Job drawing, mm, ordinate dimensions from the low corner. One solid piece. A direction names the side the tool comes from. Round coordinates to 2 decimals unless told otherwise and drop trailing zeros. Loops run counter-clockwise (first coordinate to the right, second up) from the corner with the lowest first, then second, coordinate; pieces in that order, holes last. Notation, with made-up numbers: (33.5, 37) - (57.5, 37) arc R17 cw to (57.5, 54) - close; hole circle Ø1 at (27.25, 16). An arc over 180 degrees is marked (long way). One line per question, with ' | ' between items. Start each with the question number.
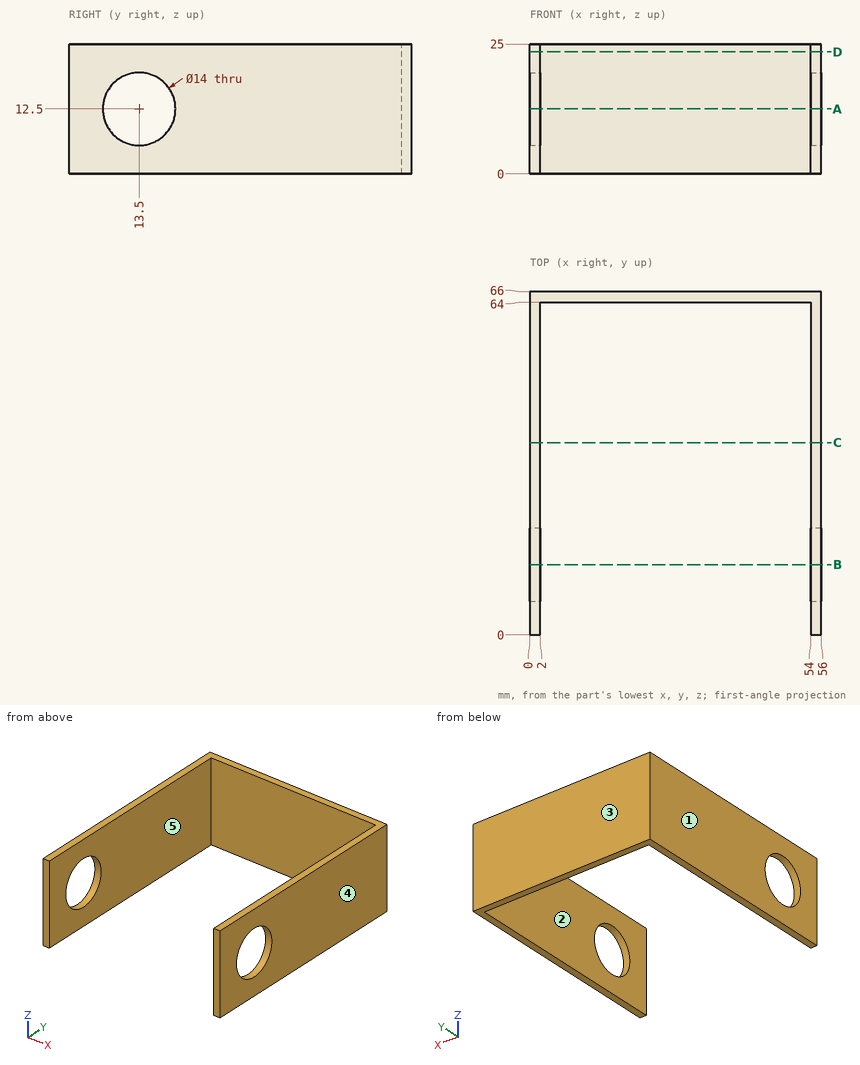
1) Saw through at B-B on y = 13.5. Write the cut outline in (x, z), and give its area (3 significant figures).
2) Tool access for the marked faces 1 and 2: list every direction of +Z, -Z, +X, -X, +Y, -Y with a clear straight run to the whole face (end or side of a thin tool).
3) Saw through at C-C on y = 37. Write the cut outline in (x, z).
4) Saw through at D-D on z = 23.5. Write the cut outline in (x, y), and give its area (3 significant figures).
5) Saw through at A-A on z = 12.5. Write the cut outline in (x, y), and give its area (3 significant figures).
6) Wall check: line 1 (X direction, y = 34, z = 20); line 2 (Z direction, x = 54.65, y = 13.5); line 3 (Y direction, x = 34.5, z = 3.5). Give the ranges that are in metal, low to high. Write a range as [from, to].
7) Drop a flat-ended pin along its axis: pin 1 (7.5 mm diameter, centred on x = 37, z = 16.5, fed in from -Y). Give the stop position or say it passes through.
8) Two-plate mould, pull along X, no slides. Class the marked faces 3, 4 and 5: +X half, -X half, draft (parallel to the pull), parting line (faces both ways), or undercut.
Answer key:
1) outline: (0, 0) - (2, 0) - (2, 5.5) - (0, 5.5) - close; (0, 19.5) - (2, 19.5) - (2, 25) - (0, 25) - close; (54, 0) - (56, 0) - (56, 5.5) - (54, 5.5) - close; (54, 19.5) - (56, 19.5) - (56, 25) - (54, 25) - close | area: 44.0 mm²
2) face 1: +Z, -Z, -X, +Y, -Y | face 2: +Z, -Z, -Y
3) outline: (0, 0) - (2, 0) - (2, 25) - (0, 25) - close; (54, 0) - (56, 0) - (56, 25) - (54, 25) - close
4) outline: (0, 0) - (2, 0) - (2, 64) - (54, 64) - (54, 0) - (56, 0) - (56, 66) - (0, 66) - close | area: 368 mm²
5) outline: (0, 0) - (2, 0) - (2, 6.5) - (0, 6.5) - close; (0, 20.5) - (2, 20.5) - (2, 64) - (54, 64) - (54, 20.5) - (56, 20.5) - (56, 66) - (0, 66) - close; (54, 0) - (56, 0) - (56, 6.5) - (54, 6.5) - close | area: 312 mm²
6) line 1: [0, 2], [54, 56] | line 2: [0, 5.5], [19.5, 25] | line 3: [64, 66]
7) pin 1: y = 64
8) face 3: draft | face 4: +X half | face 5: undercut
